Design review of the part built by this model. Coordinates are the model's own, in mm. A direction names the side the tool comes from. Give positions to 0.01 mm unless a question says otherwise; leave off trailing zeros. Loops run counter-clockwise (first coordinate to the right, second up) from the corner with the lowest first, then second, coordinate; pieces in that order, holes last. Notation, with made-up numbers: M 13.5,61.5 L 71.5,61.5 A27 ccw 71.5,83.5 Z; hole C 32.25,76.5 d4. An arc over 180 degrees is marked long. Use one line per item in the form item = value. Start each with the question number.
Autodesk Inventor part; units mm, degrees
ref_plane "YZ Plane" through (0, 0, 0) normal (1, 0, 0) x (0, 1, 0)
ref_plane "XZ Plane" through (0, 0, 0) normal (0, 1, 0) x (-1, 0, 0)
ref_plane "XY Plane" through (0, 0, 0) normal (0, 0, 1) x (1, 0, 0)
sketch "Schizzo1" plane through (0, 0, 0) normal (0, 0, 1) x (1, 0, 0)
  line L0 (10, -10) -> (-10, -10)
  line L1 (-10, -10) -> (-10, 10)
  line L2 (-10, 10) -> (10, 10)
  line L3 (10, 10) -> (10, -10)
  line L4 (9, 9) -> (-9, 9)
  line L5 (-9, 9) -> (-9, -9)
  line L6 (-9, -9) -> (9, -9)
  line L7 (9, -9) -> (9, 9)
  point P0 (0, 0)
  point P1 (0, 0)
  dimension "d0" = 20
  dimension "d1" = 1
extrude "Estrusione1" add sketch "Schizzo1" against normal blind 153
sketch "Schizzo8" plane through (10, -10, 0) normal (1, 0, 0) x (0, 0, -1)
  circle A0 centre (126, 10) radius 2.75
  circle A1 centre (27, 10) radius 2.95
  circle A2 centre (126, 10) radius 2.75
  circle A3 centre (27, 10) radius 2.95
  point P0 (0, 10)
hole "Foro7" at (10, 0, -126) at (10, 0, -27) direction (-1, 0, 0) diameter 5.9 end through all
sketch "Schizzo9" plane through (-10, 10, 0) normal (0, 1, 0) x (1, 0, 0)
  circle A0 centre (10, 13) radius 2.95
  circle A1 centre (10, 140) radius 2.75
  circle A2 centre (10, 13) radius 2.95
  circle A3 centre (10, 140) radius 2.75
  point P0 (10, 0)
hole "Foro8" at (0, 10, -13) at (0, 10, -140) direction (0, -1, 0) diameter 5.9 end through all
properties part number "4_barra" material "Alluminio D=2.26"
Q1. Take a section at D-D on z = -59. Give the boundary of the cut face in (x, y), plus the area to 3 significant figures.
Q2. For faces 1 (the cylindrical face through (9.493, 1.13, -29.725)), 2 (the flat face through (0, 9, -75)), list the 3-axis set-ups (+Z, -Z, +X, -X, +Y, -Y) from which the entire face can be reached by the end or side of a thin tool; tool diameter is ignored.
Q3. Clearance check with a flat-ended pin moving along its axis: pin 1 Ø3.5 at (y, z) = (0, -126) entering from -X. State where the tip first meets the part, or that it passes through.
Q4. Take a section at B-B on x = 0. Give the boundary of the cut face in (y, z), plus the area to 3 significant figures.
Q5. Wall thickness on probe 1 along Z at (x, y) = (0, 9.6); probe 2 along Z at (x, y) = (-9.45, 0); probe 3 along Y at (x, z) = (5.25, -29): over which ranges is each line inside the solid? List them lowest first.
Q6. Take a section at C-C on y = 7. Give the boundary of the cut face in (x, z), plus the area to 3 significant figures.
Q7. Take a section at A-A on z = -140. Give the boundary of the cut face in (x, y).
Q8. The part is to be moulded in two halves that separate along Y. For faces 3 (the flat face through (-9, 0, -75)), 4 (the cylindrical face through (-0.13, 9.493, -15.947)), 5 (the flat face through (0, 10, -75)), 6 (the flat face through (0, -9, -75)), say which applies: pulls with the +Y half, pulls with the -Y half, needs draft (parallel to the pull), parting line crosses it, or undercut.
Response values:
q1.outline = M -10,-10 L 10,-10 L 10,10 L -10,10 Z; hole M -9,-9 L 9,-9 L 9,9 L -9,9 Z
q1.area = 76.0 mm^2
q2.face_1 = +X, -X
q2.face_2 = +Z, -Z
q3.pin_1 = through
q4.outline = M -10,-153 L -9,-153 L -9,-142.95 L -10,-142.95 Z; M -10,-137.05 L -9,-137.05 L -9,-15.95 L -10,-15.95 Z; M -10,-10.05 L -9,-10.05 L -9,0 L -10,0 Z; M 9,-153 L 10,-153 L 10,-142.95 L 9,-142.95 Z; M 9,-137.05 L 10,-137.05 L 10,-15.95 L 9,-15.95 Z; M 9,-10.05 L 10,-10.05 L 10,0 L 9,0 Z
q4.area = 282 mm^2
q5.probe_1 = -153 to -142.95, -137.05 to -15.95, -10.05 to 0
q5.probe_2 = -153 to -128.95, -123.05 to -29.95, -24.05 to 0
q5.probe_3 = -10 to -9, 9 to 10
q6.outline = M -10,-153 L -9,-153 L -9,0 L -10,0 Z; M 9,-153 L 10,-153 L 10,0 L 9,0 Z
q6.area = 306 mm^2
q7.outline = M -10,-10 L -2.95,-10 L -2.95,-9 L -9,-9 L -9,9 L -2.95,9 L -2.95,10 L -10,10 Z; M 2.95,-10 L 10,-10 L 10,10 L 2.95,10 L 2.95,9 L 9,9 L 9,-9 L 2.95,-9 Z
q8.face_3 = undercut
q8.face_4 = needs draft
q8.face_5 = pulls with the +Y half
q8.face_6 = undercut
